```python
from build123d import *

# Parameters (mm, degrees)
F0_R     = 3.65
F1_DEPTH = 13.3
F3_DEPTH = 11
F4_R     = 6.65
F6_DEPTH = 25
F7_R     = 0.5
F8_SIZE  = 0.5


with BuildPart() as f1:
    # F0 (on Top) → F1 (new body)
    with BuildSketch(Plane.XY):
        with BuildLine():
            ThreePointArc((0, -6.65), (6.65, 0), (0, 6.65))
            Line((0, 6.65), (-16.45, 6.65))
            Line((-16.45, 6.65), (-16.45, -6.65))
            Line((-16.45, -6.65), (0, -6.65))
        make_face()
        with Locations((-9.8, 0)):
            Circle(F0_R, mode=Mode.SUBTRACT)
        Circle(F0_R, mode=Mode.SUBTRACT)
        with Locations((-9.8, 0)):
            Circle(F0_R)
    extrude(amount=F1_DEPTH)

    # F2 (on face) → F3 (cut)
    with BuildSketch(Plane.XZ.offset(6.65)):
        with BuildLine():
            Line((-9.9, 10.7491869112), (-11.675, 9.7243901834))
            ThreePointArc((-11.675, 9.7243901834), (-9.9, 3.1), (-8.125, 9.7243901834))
            Line((-8.125, 9.7243901834), (-9.9, 10.7491869112))
        make_face()
    extrude(amount=-F3_DEPTH, mode=Mode.SUBTRACT)

    # F4
    f4_edges = [f1.edges().sort_by_distance(p)[0] for p in [
        (-16.45, 0, 13.3),
    ]]
    fillet(f4_edges, radius=F4_R)

    # F5 (on face) → F6 (cut)
    with BuildSketch(Plane.XZ.offset(6.65)):
        with BuildLine():
            Line((-16.45, 0), (-12.5545201898, 0))
            Line((-12.5545201898, 0), (-14.5022600949, 1.9477399051))
            ThreePointArc((-14.5022600949, 1.9477399051), (-15.9437988912, 4.1051551748), (-16.45, 6.65))
            Line((-16.45, 6.65), (-16.45, 0))
        make_face()
    extrude(amount=-F6_DEPTH, mode=Mode.SUBTRACT)

    # F7
    f7_edges = [f1.edges().sort_by_distance(p)[0] for p in [
        (-4.9, -6.65, 13.3),
        (6.65, 0, 13.3),
        (-4.9, 6.65, 13.3),
        (-15.943799, 6.65, 9.194845),
        (-12.55452, 0, 0),
        (-13.52839, -6.65, 0.97387),
        (-6.27726, -6.65, 0),
        (6.65, 0, 0),
        (-15.943799, -6.65, 9.194845),
        (-6.27726, 6.65, 0),
        (-13.52839, 6.65, 0.97387),
    ]]
    fillet(f7_edges, radius=F7_R)

    # F8
    f8_edges = [f1.edges().sort_by_distance(p)[0] for p in [
        (-9.9, -6.65, 3.1),
        (-3.65, 0, 13.3),
        (-3.65, 0, 0),
        (-9.0125, -6.65, 10.236789),
        (-10.7875, -6.65, 10.236789),
    ]]
    chamfer(f8_edges, length=F8_SIZE)


solid = f1.part
```
Geometry check sheet. Reference: the model listing, model coordinates, mm. A direction names the side the tool comes from. Round coordinates to 2 decimals unless told otherwise and drop trailing zeros. Loops run counter-clockwise (first coordinate to the right, second up) from the corner with the lowest first, then second, coordinate; pieces in that order, holes last. Notation, with made-up numbers: (61, -21) -> (89, -21) arc R22 cw to (89, -2) -> close; hole circle Ø9 at (85.5, -36.75). An arc over 180 degrees is marked (long way). Use a Markdown table: item, result.
(1) Sectioned sample at A-A (y = 0). Enter the section's corners in (x, z) (3 decimals).
Calculated:
| item | result |
|---|---|
| outline | (-14.502, 1.948) -> (-12.701, 0.146) arc R0.5 ccw to (-12.347, 0) -> (-4.15, 0) -> (-3.65, 0.5) -> (-3.65, 12.8) -> (-4.15, 13.3) -> (-9.8, 13.3) arc R6.65 ccw to start; (3.65, 0.5) -> (4.15, 0) -> (6.15, 0) arc R0.5 ccw to (6.65, 0.5) -> (6.65, 12.8) arc R0.5 ccw to (6.15, 13.3) -> (4.15, 13.3) -> (3.65, 12.8) -> close; hole (-11.675, 9.724) arc R3.55 ccw (long way) to (-8.125, 9.724) -> (-9.9, 10.749) -> close |
(2) Go/stop test with flat-tipped pins: P1, Ø1.5, axis at y = 1, z = 8, coming from the +X side; P2, Ø1, axis at x = 1.5, z = 3, coming from the -Y side; P3, Ø3.5, axis at x = -9, z = 7.5, coming from the -Y side. Record where each tip stops, or that it passes through.
Calculated:
| item | result |
|---|---|
| P1 | x = 6.65 |
| P2 | y = -6.57 |
| P3 | y = 4.35 |
(3) Set-up check for faces 4 (the flat face through (-10.772, -6.396, 10.531)), 5 (the cylindrical face through (-13.48, 6.51, 1.14)): record each of +Z, -Z, +X, -X, +Y, -Y from which the full face is reachable in a straight line by a thin tool's end or side.
Calculated:
| item | result |
|---|---|
| face 4 | -Y |
| face 5 | -Z, -X, +Y |
(4) Scan lines: probe 1 along Y at (x, z) = (0, 7.25); probe 2 along X at (y, z) = (-2.75, 6.65); probe 3 along X at (y, z) = (-2, 3.5). Record each from-to range of solid material in increasing order.
Calculated:
| item | result |
|---|---|
| probe 1 | -6.65 to -3.65, 3.65 to 6.65 |
| probe 2 | -16.45 to -13.45, -6.35 to -2.4, 2.4 to 6.05 |
| probe 3 | -15.66 to -11.54, -8.26 to -3.05, 3.05 to 6.34 |
(5) Mould release check, pull along X, two halves, no side actions. Record for faces 1 (the cylindrical face through (6.65, -0.15, 6.56)), 2 (the cylindrical face through (-10, -1, 3.1)), 3 (the flat face through (-5, 0, 13.3)): released by +X, released by -X, zero draft, split by the parting line, or undercut.
Calculated:
| item | result |
|---|---|
| face 1 | released by +X |
| face 2 | undercut |
| face 3 | zero draft |
